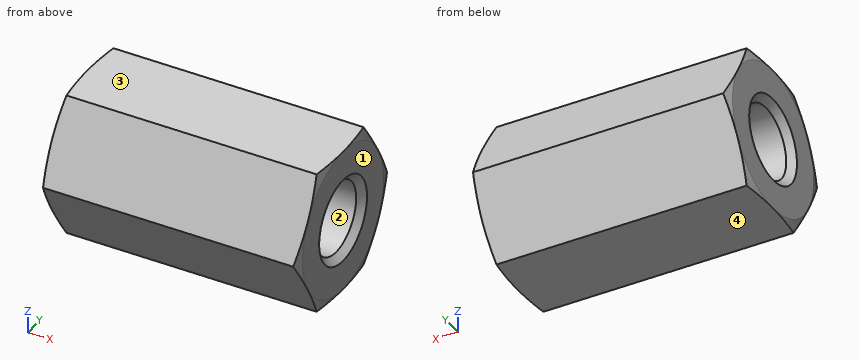
Autodesk Inventor part; units mm, degrees
ref_plane "IP1_XY" through (0, 0, 0) normal (1, 0, 0) x (0, 0, -1)
ref_plane "IP1_YZ" through (0, 0, 0) normal (0, 0, -1) x (0, 1, 0)
ref_plane "IP1_ZX" through (0, 0, 0) normal (0, 1, 0) x (1, 0, 0)
sketch "Sketch_1" plane through (0, 0, 0) normal (0, 0, 1) x (1, 0, 0)
  line L0 (30, 0) -> (0, 0)
  line L1 (0, 0) -> (0, 10.2)
  line L2 (0, 10.2) -> (30, 10.2)
  line L3 (30, 10.2) -> (30, 0)
  line L4 (30, 0) -> (0, 0)
revolve "Revolution1" add sketch "Sketch_1" angle 360 about axis through (30, 0, 0) along (-1, 0, 0)
sketch "Sketch_4" plane through (0, 0, 0) normal (0, 0, 1) x (1, 0, 0)
  line L0 (30, 0) -> (0, 0)
  line L1 (0, 8.5) -> (0.4555, 10.2)
  line L2 (0.4555, 10.2) -> (0, 10.2)
  line L3 (0, 10.2) -> (0, 8.5)
revolve "Revolution2" cut sketch "Sketch_4" angle 360 about axis through (30, 0, 0) along (1, 0, 0)
sketch "Sketch_5" plane through (0, 0, 0) normal (0, 0, 1) x (1, 0, 0)
  line L0 (30, 0) -> (0, 0)
  line L1 (29.5445, 10.2) -> (30, 8.5)
  line L2 (30, 8.5) -> (30, 10.2)
  line L3 (30, 10.2) -> (29.5445, 10.2)
revolve "Revolution3" cut sketch "Sketch_5" angle 360 about axis through (30, 0, 0) along (1, 0, 0)
sketch "Sketch_3" plane through (0, 0, 0) normal (0, 0, 1) x (1, 0, 0)
  line L0 (30, 0) -> (0, 0)
  line L1 (0, 0) -> (0, 5)
  line L2 (0, 5) -> (0.812, 4.188)
  line L3 (0.812, 4.188) -> (29.188, 4.188)
  line L4 (29.188, 4.188) -> (30, 5)
  line L5 (30, 5) -> (30, 0)
  line L6 (30, 0) -> (0, 0)
revolve "Revolution4" cut sketch "Sketch_3" angle 360 about axis through (30, 0, 0) along (1, 0, 0)
thread "Thread1"
sketch "Sketch_2" plane through (0, 0, 0) normal (1, 0, 0) x (0, 1, 0)
  line L0 (34, 34) -> (-34, 34)
  line L1 (-34, 34) -> (-34, -34)
  line L2 (-34, -34) -> (34, -34)
  line L3 (34, -34) -> (34, 34)
  line L4 (-4.9075, 8.5) -> (-9.815, 0)
  line L5 (-9.815, 0) -> (-4.9075, -8.5)
  line L6 (-4.9075, -8.5) -> (4.9075, -8.5)
  line L7 (4.9075, -8.5) -> (9.815, 0)
  line L8 (9.815, 0) -> (4.9075, 8.5)
  line L9 (4.9075, 8.5) -> (-4.9075, 8.5)
extrude "Extrusion1" cut sketch "Sketch_2" along normal mid plane 62
ref_plane "IP1_XY" through (0, 0, 0) normal (1, 0, 0) x (0, 0, -1)
ref_plane "IP1_YZ" through (0, 0, 0) normal (0, 0, -1) x (0, 1, 0)
ref_plane "IP1_ZX" through (0, 0, 0) normal (0, 1, 0) x (1, 0, 0)
ref_plane "IP2_XY" through (30, 0, 0) normal (1, 0, 0) x (0, 0, -1)
ref_plane "IP2_YZ" through (30, 0, 0) normal (0, 0, -1) x (0, 1, 0)
ref_plane "IP2_ZX" through (30, 0, 0) normal (0, 1, 0) x (1, 0, 0)
properties part number "Hexagon nut DIN 6334 M10 51103.100.040(High)"
The model under review builds one solid part; all positions refer to its coordinate system, in mm. Face numbers are marked on the shaded views. Give positions to 0.01 mm unless a question says otherwise; leave off trailing zeros. Write each loop counter-clockwise with the first axis right and the second up, starting at its lowest first coordinate (ties: lowest second). Pieces come first, ordered by that corner, then holes. Notation, with made-up numbers: M 11,-38 L 60,-38 A27 ccw 60,0 Z; hole C 36.25,57.5 d5. An arc over 180 degrees is marked long. Write item = value, one per line. Start each with the question number.
Q1. Clearance check with flat-ended pins moving along their axes: pin 1 (8 mm diameter, centred on x = 19.5, z = -6, fed in from +Y); pin 2 (10 mm diameter, centred on x = 13, z = -6.5, fed in from +Y); pin 3 (6.5 mm diameter, centred on y = 0, z = 0, fed in from +X); pin 4 (4 mm diameter, centred on y = 2, z = -1.5, fed in from +X). State where each tip first meets the part, or that it passes through.
Q2. Mouldability with a two-part tool opening along Z and no side actions: class the marked faces 1, 2, 3 and 4 as released by +Z, released by -Z, zero draft, split by the parting line, or undercut.
Q3. We need section A-A (x = 14). State the section outline as (y, z) points (1 decimal), plus the area to 3 significant figures.
Q4. For line 1 (Z direction, x = 12.5, y = 0); line 2 (Y direction, x = 20.5, z = -1.75); line 3 (Y direction, x = 22, z = 1), list the stretches that pass through material, from the lowest coordinate up.
Result set:
q1.pin_1 = 8.66
q1.pin_2 = 8.95
q1.pin_3 = through
q1.pin_4 = 29.5
q2.face_1 = zero draft
q2.face_2 = undercut
q2.face_3 = released by +Z
q2.face_4 = released by -Z
q3.outline = M -9.8,0 L -4.9,-8.5 L 4.9,-8.5 L 9.8,0 L 4.9,8.5 L -4.9,8.5 Z; hole C 0,0 d8.4
q3.area = 195 mm2
q4.line_1 = -8.5 to -4.19, 4.19 to 8.5
q4.line_2 = -8.8 to -3.8, 3.8 to 8.8
q4.line_3 = -9.24 to -4.07, 4.07 to 9.24
